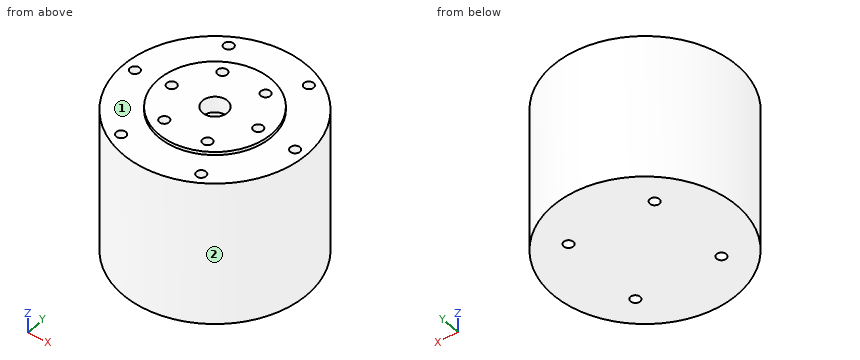
```python
from build123d import *

# Parameters (mm, degrees)
SKETCH_1_R          = 28.5
EXTRUDE_1_DEPTH     = 45
SKETCH_2_R          = 1.5
CUT_EXTRUDE_1_DEPTH = 4
SKETCH_3_R          = 1.5
CUT_EXTRUDE_2_DEPTH = 5
SKETCH_4_R          = 17.5
EXTRUDE_2_DEPTH     = 1
SKETCH_5_R          = 1.5
SKETCH_5_R_2        = 3.876309497
CUT_EXTRUDE_3_DEPTH = 5


with BuildPart() as part:
    # 草图1 → 凸台-拉伸1 (new body)
    with BuildSketch(Plane.XY):
        Circle(SKETCH_1_R)
    extrude(amount=EXTRUDE_1_DEPTH)

    # 草图2 → 切除-拉伸1 (cut)
    with BuildSketch(Plane(origin=(0, 0, 0), x_dir=(-1, 0, 0), z_dir=(0, 0, -1))):
        with Locations((13.435028843, -13.435028843)):
            Circle(SKETCH_2_R)
        with Locations((-13.435028843, -13.435028843)):
            Circle(SKETCH_2_R)
        with Locations((-13.435028843, 13.435028843)):
            Circle(SKETCH_2_R)
        with Locations((13.435028843, 13.435028843)):
            Circle(SKETCH_2_R)
    extrude(amount=-CUT_EXTRUDE_1_DEPTH, mode=Mode.SUBTRACT)

    # 草图3 → 切除-拉伸2 (cut)
    with BuildSketch(Plane.XY.offset(45)):
        with Locations((-12.5, -21.650635095)):
            Circle(SKETCH_3_R)
        with Locations((-12.5, 21.650635095)):
            Circle(SKETCH_3_R)
        with Locations((12.5, 21.650635095)):
            Circle(SKETCH_3_R)
        with Locations((12.5, -21.650635095)):
            Circle(SKETCH_3_R)
        with Locations((-25, 0)):
            Circle(SKETCH_3_R)
        with Locations((25, 0)):
            Circle(SKETCH_3_R)
    extrude(amount=-CUT_EXTRUDE_2_DEPTH, mode=Mode.SUBTRACT)

    # 草图4 → 凸台-拉伸2 (add)
    with BuildSketch(Plane.XY.offset(45)):
        Circle(SKETCH_4_R)
    extrude(amount=EXTRUDE_2_DEPTH)

    # 草图5 → 切除-拉伸3 (cut)
    with BuildSketch(Plane.XY.offset(46)):
        with Locations((13.5, 0)):
            Circle(SKETCH_5_R)
        with Locations((-13.5, 0)):
            Circle(SKETCH_5_R)
        with Locations((6.75, 11.691342951)):
            Circle(SKETCH_5_R)
        with Locations((-6.75, 11.691342951)):
            Circle(SKETCH_5_R)
        with Locations((-6.75, -11.691342951)):
            Circle(SKETCH_5_R)
        with Locations((6.75, -11.691342951)):
            Circle(SKETCH_5_R)
        Circle(SKETCH_5_R_2)
    extrude(amount=-CUT_EXTRUDE_3_DEPTH, mode=Mode.SUBTRACT)


solid = part.part
```
Here's how the part is built. I have some questions about the finished solid (model axes, mm). Face numbers are marked on the shaded views. A direction names the side the tool comes from. Coordinates: 2 decimals unless noted, no trailing zeros. Order: outer loops, then holes, each group sorted by start corner. A loop starts at its lowest first (then second) coordinate and runs counter-clockwise, first axis right, second up. Notation, with made-up numbers: (-17.5, 53) - (0.5, 53) arc R13 cw to (0.5, 68) - close; hole circle Ø6 at (48.25, 19.5). An arc over 180 degrees is marked (long way). One line per question, with ' | ' between items.
(1) Suppose I cut it at B-B on x = 0.5. List the corners of the cut face in (y, z) for me, and give its area (3 significant figures).
Report:
outline: (-28.5, 0) - (28.5, 0) - (28.5, 45) - (17.49, 45) - (17.49, 46) - (3.84, 46) - (3.84, 41) - (-3.84, 41) - (-3.84, 46) - (-17.49, 46) - (-17.49, 45) - (-28.5, 45) - close | area: 2,560 mm2
(2) If I drill on L1, parallel to Y at x = 0, z = 44.3; L2, parallel to Y at x = 6, z = 44; L3, parallel to Z at x = 25, y = -8, over which ranges is the centre line in solid material (lowest first)?
Report:
L1: y = -28.5 to -3.88, 3.88 to 28.5 | L2: y = -27.86 to -12.99, -10.39 to 10.39, 12.99 to 27.86 | L3: z = 0 to 45
(3) Will these pins go through, and if not, where does the flat tip stop? pin 1 (2 mm diameter, centred on y = -4, z = 20, fed in from -X); pin 2 (2.5 mm diameter, centred on x = -6.75, y = -11.69, fed in from +Z); pin 3 (1.5 mm diameter, centred on y = 21, z = 14, fed in from +X).
Report:
pin 1: stops at x = -28.34 | pin 2: stops at z = 41 | pin 3: stops at x = 20.05
(4) Suppose I cut it at A-A on y = 0. List the corners of the cut face in (x, z) for me.
Report:
outline: (-28.5, 0) - (28.5, 0) - (28.5, 45) - (26.5, 45) - (26.5, 40) - (23.5, 40) - (23.5, 45) - (17.5, 45) - (17.5, 46) - (15, 46) - (15, 41) - (12, 41) - (12, 46) - (3.88, 46) - (3.88, 41) - (-3.88, 41) - (-3.88, 46) - (-12, 46) - (-12, 41) - (-15, 41) - (-15, 46) - (-17.5, 46) - (-17.5, 45) - (-23.5, 45) - (-23.5, 40) - (-26.5, 40) - (-26.5, 45) - (-28.5, 45) - close
(5) Suppose I cut it at C-C on z = 36. List the corners of the cut face in (x, y) for me, and give its area (3 significant figures).
Report:
outline: circle Ø57 at (0, 0) | area: 2,550 mm2
(6) Suppose I cut it at D-D on x = 25. List the corners of the cut face in (y, z) for me, and give its area (3 significant figures).
Report:
outline: (-13.68, 0) - (13.68, 0) - (13.68, 45) - (1.5, 45) - (1.5, 40) - (-1.5, 40) - (-1.5, 45) - (-13.68, 45) - close | area: 1,220 mm2
(7) For the marked faces 1 and 2, which set-ups out of +Z, -Z, +X, -X, +Y, -Y let a thin tool reach every point of the face, with its end or its side?
Report:
face 1: +Z | face 2: +Z, -Z
